Here's how the part is built. I have some questions about the finished solid (model axes, mm). A direction names the side the tool comes from. Round coordinates to 2 decimals unless told otherwise and drop trailing zeros. Order: outer loops, then holes, each group sorted by start corner. A loop starts at its lowest first (then second) coordinate and runs counter-clockwise, first axis right, second up. Notation, with made-up numbers: (13.25, -6) -> (29.25, -6) arc R19 cw to (29.25, -2) -> close; hole circle Ø5 at (-33, -32.75). An arc over 180 degrees is marked (long way). Use a Markdown table: item, result. Add a question column.
(1) If I drill on probe 1 along Y at (x, z) = (0, 5.5); probe 2 along Y at (x, z) = (4.75, 6); probe 3 along X at (y, z) = (-7.5, 4.75), over which ranges is the centre line in solid material (lowest first)?
(2) I want a section at B-B, the plane z = 4. Please give me the cut outline in (x, y), then the cut area to 3 significant figures.
(3) I want a section at C-C, the plane y = 10.5. Please give me the cut outline in (x, z).
(4) I want a section at A-A, the plane x = 4. Please give me the cut outline in (y, z), then the cut area to 3 significant figures.
(5) On a 3-axis mill with a long thin cutter (end or side, diameter ignored), from which of +Z, -Z, +X, -X, +Y, -Y can I reach the whole of each face in a straight line? I mean faces 1 (the face through (6, 13.8, 5)), 2 (the face through (0, 11.5, 5)), 3 (the face through (-6, -13.8, 5)), 4 (the face through (-6, 13.8, 5)), 5 (the face through (6, -13.8, 5)). Say none if no direction works.
(6) I'm going to push flat-ended pins straight in: P1, Ø3, axis at x = -5.5, z = 5.5, coming from the +Y side; P2, Ø2, axis at x = -2.5, z = 2, coming from the -Y side; P3, Ø4.5, axis at x = -6.5, z = 4.5, coming from the -Y side; P4, Ø1.5, axis at x = 0.5, z = 2.5, coming from the +Y side. Where does each tip first touch, or does it pass through?
(7) I want a section at D-D, the plane x = 0. Please give me the cut outline in (y, z), then the cut area to 3 significant figures.
(8) Thinking about a two-plate mould opening in X: for faces 6 (the face through (6, 0, 5)), 7 (the face through (-8.5, 0, 5)), 8 (the face through (-6.3, 0.1, 9.3)), which applies, pulls with the +X half, pulls with the -X half, needs draft (parallel to the pull), parting line crosses it, or undercut?
from build123d import *

# Parameters (mm, degrees)
SKETCH1_R           = 1.3
SKETCH1_W           = 12
SKETCH1_H           = 23
BOSS_EXTRUDE1_DEPTH = 9.3


with BuildPart() as part:
    # Sketch1 → Boss-Extrude1 (new body)
    with BuildSketch(Plane.XY):
        with BuildLine():
            Line((-3, 13.8), (-8.5, 13.8))
            Line((-8.5, 13.8), (-8.5, -13.8))
            Line((-8.5, -13.8), (-3, -13.8))
            ThreePointArc((-3, -13.8), (0, -16.8), (3, -13.8))
            Line((3, -13.8), (8.5, -13.8))
            Line((8.5, -13.8), (8.5, 13.8))
            Line((8.5, 13.8), (3, 13.8))
            ThreePointArc((3, 13.8), (0, 16.8), (-3, 13.8))
        make_face()
        with Locations((0, 13.8)):
            Circle(SKETCH1_R, mode=Mode.SUBTRACT)
        with Locations((0, -13.8)):
            Circle(SKETCH1_R, mode=Mode.SUBTRACT)
        Rectangle(SKETCH1_W, SKETCH1_H, mode=Mode.SUBTRACT)
    extrude(amount=BOSS_EXTRUDE1_DEPTH)


solid = part.part
Taken from the geometry:
| question | item | result |
|---|---|---|
| 1 | probe 1 | y = -16.8 to -15.1, -12.5 to -11.5, 11.5 to 12.5, 15.1 to 16.8 |
| 1 | probe 2 | y = -13.8 to -11.5, 11.5 to 13.8 |
| 1 | probe 3 | x = -8.5 to -6, 6 to 8.5 |
| 2 | outline | (-8.5, -13.8) -> (-3, -13.8) arc R3 ccw to (3, -13.8) -> (8.5, -13.8) -> (8.5, 13.8) -> (3, 13.8) arc R3 ccw to (-3, 13.8) -> (-8.5, 13.8) -> close; hole (-6, -11.5) -> (6, -11.5) -> (6, 11.5) -> (-6, 11.5) -> close; hole circle Ø2.6 at (0, -13.8); hole circle Ø2.6 at (0, 13.8) |
| 2 | area | 211 mm2 |
| 3 | outline | (-8.5, 0) -> (-6, 0) -> (-6, 9.3) -> (-8.5, 9.3) -> close; (6, 0) -> (8.5, 0) -> (8.5, 9.3) -> (6, 9.3) -> close |
| 4 | outline | (-13.8, 0) -> (-11.5, 0) -> (-11.5, 9.3) -> (-13.8, 9.3) -> close; (11.5, 0) -> (13.8, 0) -> (13.8, 9.3) -> (11.5, 9.3) -> close |
| 4 | area | 42.8 mm2 |
| 5 | face 1 | +Z, -Z, +X, +Y |
| 5 | face 2 | +Z, -Z |
| 5 | face 3 | +Z, -Z, -X, -Y |
| 5 | face 4 | +Z, -Z, -X, +Y |
| 5 | face 5 | +Z, -Z, +X, -Y |
| 6 | P1 | stops at y = 13.8 |
| 6 | P2 | stops at y = -16.4 |
| 6 | P3 | stops at y = -13.8 |
| 6 | P4 | stops at y = 16.8 |
| 7 | outline | (-16.8, 0) -> (-15.1, 0) -> (-15.1, 9.3) -> (-16.8, 9.3) -> close; (-12.5, 0) -> (-11.5, 0) -> (-11.5, 9.3) -> (-12.5, 9.3) -> close; (11.5, 0) -> (12.5, 0) -> (12.5, 9.3) -> (11.5, 9.3) -> close; (15.1, 0) -> (16.8, 0) -> (16.8, 9.3) -> (15.1, 9.3) -> close |
| 7 | area | 50.2 mm2 |
| 8 | face 6 | undercut |
| 8 | face 7 | pulls with the -X half |
| 8 | face 8 | needs draft |
